Here's the drawing with two shaded views (mm, measured from the low corner). I have some questions. Give positions to 0.01 mm unless a question says otherwise; leave off trailing zeros. Write each loop counter-clockwise with the first axis right and the second up, starting at its lowest first coordinate (ties: lowest second). Pieces come first, ordered by that corner, then holes. Notation, with made-up numbers: (-1, 3.5) -> (28, 3.5) arc R19 cw to (28, 30.5) -> close; hole circle Ø7 at (66.5, 20). An arc over 180 degrees is marked (long way). Put each result on its own line as item: value. Start each with the question number.
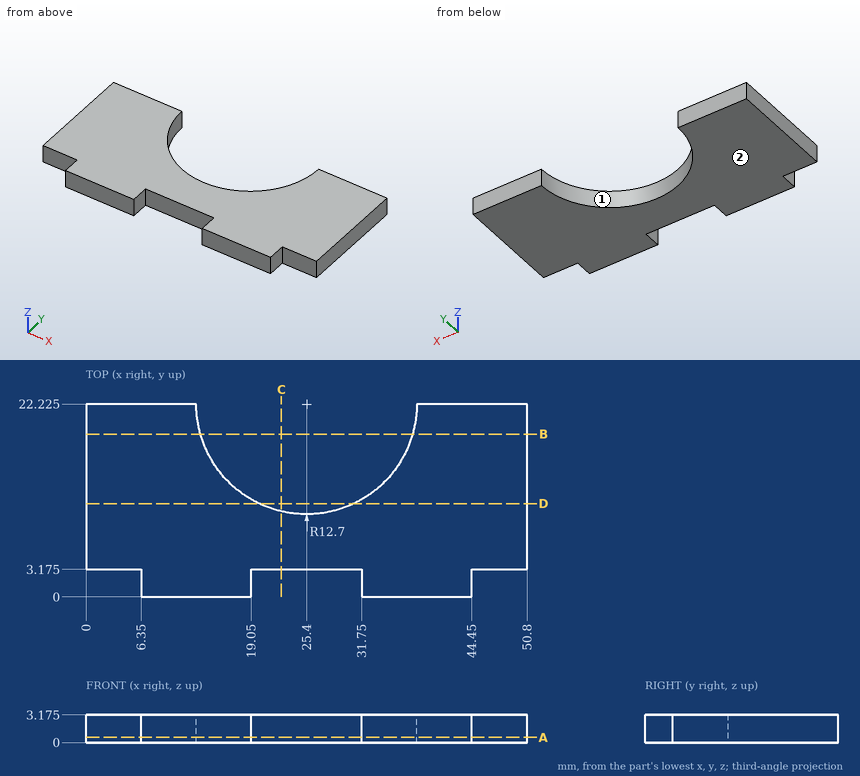
1) I need wall thicknesses on probe 1 along X at (y, z) = (3, 0.5); probe 2 along Y at (x, z) = (5, 2.15) (3 decimals); probe 3 along X at (y, z) = (20, 1.6). Which ranges of each line are inside material? Lowest first, please.
2) I want a section at A-A, the plane z = 0.6. Write out the boundary of the cut face in (x, y) (3 decimals).
3) Thinking about a two-plate mould opening in X: for the marked faces 1 and 2, which applies, released by +X, released by -X, zero draft, split by the parting line, or undercut?
4) I want a section at B-B, the plane y = 18.75. Write out the boundary of the cut face in (x, z) (3 decimals), and give its area (3 significant figures).
5) I want a section at C-C, the plane x = 22.5. Write out the boundary of the cut face in (y, z) (3 decimals), and give its area (3 significant figures).
6) I'm going to push flat-ended pins straight in: pin 1 Ø1.6 at (y, z) = (1.5, 2) entering from -X; pin 2 Ø1.6 at (y, z) = (1, 1.5) entering from +X. Where does each tip first touch, or does it pass through?
7) I want a section at D-D, the plane y = 10.75. Write out the boundary of the cut face in (x, z) (3 decimals).
Established:
1. probe 1: x = 6.35 to 19.05, 31.75 to 44.45
1. probe 2: y = 3.175 to 22.225
1. probe 3: x = 0 to 12.9, 37.9 to 50.8
2. outline: (0, 3.175) -> (6.35, 3.175) -> (6.35, 0) -> (19.05, 0) -> (19.05, 3.175) -> (31.75, 3.175) -> (31.75, 0) -> (44.45, 0) -> (44.45, 3.175) -> (50.8, 3.175) -> (50.8, 22.225) -> (38.1, 22.225) arc R12.7 cw to (12.7, 22.225) -> (0, 22.225) -> close
3. face 1: undercut
3. face 2: zero draft
4. outline: (0, 0) -> (13.185, 0) -> (13.185, 3.175) -> (0, 3.175) -> close; (37.615, 0) -> (50.8, 0) -> (50.8, 3.175) -> (37.615, 3.175) -> close
4. area: 83.7 mm2
5. outline: (3.175, 0) -> (9.861, 0) -> (9.861, 3.175) -> (3.175, 3.175) -> close
5. area: 21.2 mm2
6. pin 1: stops at x = 6.35
6. pin 2: stops at x = 44.45
7. outline: (0, 0) -> (19.958, 0) -> (19.958, 3.175) -> (0, 3.175) -> close; (30.842, 0) -> (50.8, 0) -> (50.8, 3.175) -> (30.842, 3.175) -> close
